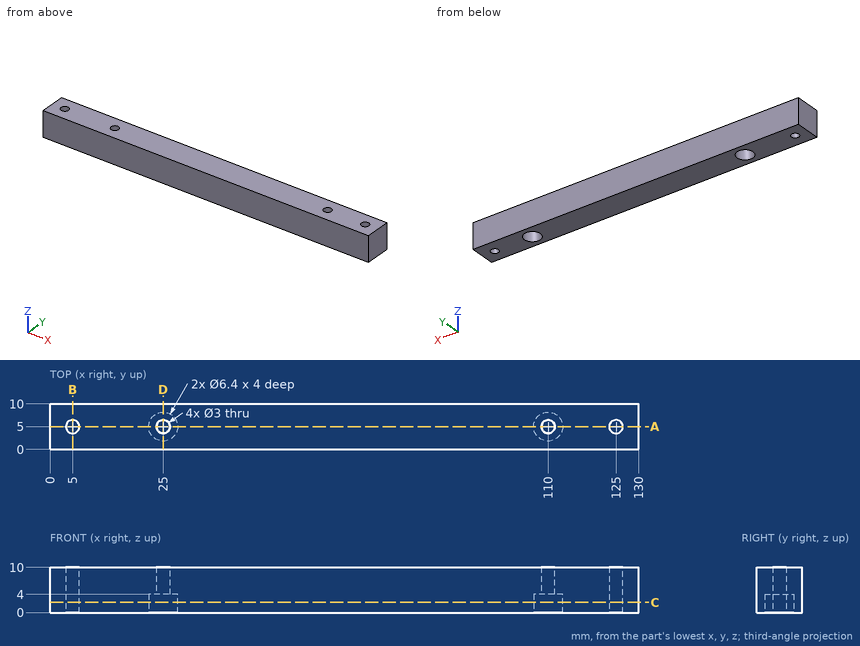
Check sheet for the drawn part. Datum: minimum x, y, z corner. Units: mm. Give positions to 0.01 mm unless a question says otherwise; leave off trailing zeros. Order: outer loops, then holes, each group sorted by start corner. A loop starts at its lowest first (then second) coordinate and runs counter-clockwise, first axis right, second up.
1. Depth check by flat-ended pin: pin 1 (1.9 mm diameter, centred on x = 110.5, y = 6, fed in from -Z); pin 2 (2.5 mm diameter, centred on x = 25, y = 5, fed in from -Z). Enter the tip coordinate at first touch or a pass-through.
Completed:
pin 1: stops at z = 4
pin 2: passes through
2. Sectioned sample at C-C (z = 2.25). Record the boundary of the cut face in (x, y).
Completed:
outline: (0, 0) - (130, 0) - (130, 10) - (0, 10) - close; hole circle Ø3 at (5, 5); hole circle Ø6.4 at (25, 5); hole circle Ø6.4 at (110, 5); hole circle Ø3 at (125, 5)
3. Sectioned sample at A-A (y = 5). Record the boundary of the cut face in (x, z), then the cut area to 3 significant figures.
Completed:
outline: (0, 0) - (3.5, 0) - (3.5, 10) - (0, 10) - close; (6.5, 0) - (21.8, 0) - (21.8, 4) - (23.5, 4) - (23.5, 10) - (6.5, 10) - close; (26.5, 4) - (28.2, 4) - (28.2, 0) - (106.8, 0) - (106.8, 4) - (108.5, 4) - (108.5, 10) - (26.5, 10) - close; (111.5, 4) - (113.2, 4) - (113.2, 0) - (123.5, 0) - (123.5, 10) - (111.5, 10) - close; (126.5, 0) - (130, 0) - (130, 10) - (126.5, 10) - close
area: 1,150 mm2
4. Scan lines: line 1 (Y direction, x = 25, z = 7.35); line 2 (X direction, y = 4.5, z = 3.75); line 3 (X direction, y = 6, z = 2.5). Record each from-to range of solid material in increasing order.
Completed:
line 1: y = 0 to 3.5, 6.5 to 10
line 2: x = 0 to 3.59, 6.41 to 21.84, 28.16 to 106.84, 113.16 to 123.59, 126.41 to 130
line 3: x = 0 to 3.88, 6.12 to 21.96, 28.04 to 106.96, 113.04 to 123.88, 126.12 to 130
5. Sectioned sample at D-D (x = 25). Record the boundary of the cut face in (y, z).
Completed:
outline: (0, 0) - (1.8, 0) - (1.8, 4) - (3.5, 4) - (3.5, 10) - (0, 10) - close; (6.5, 4) - (8.2, 4) - (8.2, 0) - (10, 0) - (10, 10) - (6.5, 10) - close
6. Sectioned sample at B-B (x = 5). Record the boundary of the cut face in (y, z), then the cut area to 3 significant figures.
Completed:
outline: (0, 0) - (3.5, 0) - (3.5, 10) - (0, 10) - close; (6.5, 0) - (10, 0) - (10, 10) - (6.5, 10) - close
area: 70.0 mm2
